Autodesk Inventor part; units mm, degrees
ref_plane "YZ Plane" through (0, 0, 0) normal (1, 0, 0) x (0, 1, 0)
ref_plane "XZ Plane" through (0, 0, 0) normal (0, 1, 0) x (-1, 0, 0)
ref_plane "XY Plane" through (0, 0, 0) normal (0, 0, 1) x (1, 0, 0)
sketch "Sketch1" plane through (0, 0, 0) normal (0, 1, 0) x (-1, 0, 0)
  line L0 (0, 0) -> (100, 0)
  line L1 (100, 0) -> (100, -100)
  line L2 (100, -100) -> (0, -100)
  line L3 (0, -100) -> (0, 0)
  dimension "d0" = 100
  dimension "d1" = 100
extrude "Extrusion1" add sketch "Sketch1" along normal blind 0.3
sketch "Sketch2" plane through (0, 0.3, 0) normal (0, 1, 0) x (1, 0, 0)
  line L0 (-100, 100) -> (-100, 0)
  line L1 (-100, 0) -> (0, 0)
  line L2 (0, 0) -> (0, 100)
  line L3 (0, 100) -> (-100, 100)
  line L4 (0, 0) -> (0, 50)
  line L5 (0, 0) -> (0, 100)
  line L6 (0, 50) -> (-50, 50)
  circle A0 centre (-50, 50) radius 1.5
  dimension "d4" = 50
  dimension "d5" = 3
extrude "Extrusion2" cut sketch "Sketch2" against normal blind 0.3 contours A0
sketch "Sketch3" plane through (0, 0.3, 0) normal (0, 1, 0) x (1, 0, 0)
  circle A0 centre (-50, 50) radius 1.5
  line L0 (-100, 100) -> (-100, 0)
  line L1 (-100, 0) -> (0, 0)
  line L2 (0, 0) -> (0, 100)
  line L3 (0, 100) -> (-100, 100)
  line L4 (-50, 50) -> (-57, 50)
  line L5 (-57, 47.5) -> (-57, 52.5) construction
  line L6 (-56.9, 47.5) -> (-56.9, 52.5)
  line L7 (-57.1, 52.5) -> (-57.1, 47.5)
  arc A1 (-57.1, 47.5) -> (-56.9, 47.5) centre (-57, 47.5) ccw
  arc A2 (-56.9, 52.5) -> (-57.1, 52.5) centre (-57, 52.5) ccw
  line L8 (-57, 50) -> (-65, 50)
  line L9 (-65, 47.5) -> (-65, 52.5) construction
  line L10 (-64.9, 47.5) -> (-64.9, 52.5)
  line L11 (-65.1, 52.5) -> (-65.1, 47.5)
  arc A3 (-65.1, 47.5) -> (-64.9, 47.5) centre (-65, 47.5) ccw
  arc A4 (-64.9, 52.5) -> (-65.1, 52.5) centre (-65, 52.5) ccw
  line L12 (-65, 50) -> (-77, 50)
  line L13 (-77, 47.5) -> (-77, 52.5) construction
  line L14 (-76.9, 47.5) -> (-76.9, 52.5)
  line L15 (-77.1, 52.5) -> (-77.1, 47.5)
  arc A5 (-77.1, 47.5) -> (-76.9, 47.5) centre (-77, 47.5) ccw
  arc A6 (-76.9, 52.5) -> (-77.1, 52.5) centre (-77, 52.5) ccw
  dimension "d8" = 7
  dimension "d9" = 2.5
  dimension "d10" = 0.2
  dimension "d11" = 8
  dimension "d12" = 2.5
  dimension "d13" = 0.2
  dimension "d14" = 12
  dimension "d15" = 2.5
  dimension "d16" = 0.2
extrude "Extrusion3" cut sketch "Sketch3" against normal blind 0.3 contours L14 A5 L15 A6 | L10 A3 L11 L12 L8 | L8 L12 L11 A4 L10 | L6 A1 L7 L8 L4 | L4 L8 L7 A2 L6
pattern_circular "Circular Pattern1" count 6 over 360 about axis through (-50, 0.3, -50) along (0, -1, 0) of "Extrusion3"
sketch "Sketch4" plane through (0, 0.3, 0) normal (0, 1, 0) x (1, 0, 0)
  line L0 (-51.3849, 42.6012) -> (-55.7151, 45.1012)
  arc A0 (-55.6151, 45.2744) -> (-55.7151, 45.1012) centre (-55.6651, 45.1878) ccw
  line L1 (-55.6151, 45.2744) -> (-51.2849, 42.7744)
  arc A1 (-51.3849, 42.6012) -> (-51.2849, 42.7744) centre (-51.3349, 42.6878) ccw
  line L2 (-55.3849, 35.673) -> (-59.7151, 38.173)
  arc A2 (-59.6151, 38.3462) -> (-59.7151, 38.173) centre (-59.6651, 38.2596) ccw
  line L3 (-59.6151, 38.3462) -> (-55.2849, 35.8462)
  arc A3 (-55.3849, 35.673) -> (-55.2849, 35.8462) centre (-55.3349, 35.7596) ccw
  arc A4 (-65.6151, 27.9539) -> (-65.7151, 27.7807) centre (-65.6651, 27.8673) ccw
  line L4 (-65.6151, 27.9539) -> (-61.2849, 25.4539)
  arc A5 (-61.3849, 25.2807) -> (-61.2849, 25.4539) centre (-61.3349, 25.3673) ccw
  line L5 (-61.3849, 25.2807) -> (-65.7151, 27.7807)
  line L6 (-44.2849, 45.1012) -> (-48.6151, 42.6012)
  arc A6 (-48.7151, 42.7744) -> (-48.6151, 42.6012) centre (-48.6651, 42.6878) ccw
  line L7 (-48.7151, 42.7744) -> (-44.3849, 45.2744)
  arc A7 (-44.2849, 45.1012) -> (-44.3849, 45.2744) centre (-44.3349, 45.1878) ccw
  line L8 (-40.2849, 38.173) -> (-44.6151, 35.673)
  arc A8 (-44.7151, 35.8462) -> (-44.6151, 35.673) centre (-44.6651, 35.7596) ccw
  line L9 (-44.7151, 35.8462) -> (-40.3849, 38.3462)
  arc A9 (-40.2849, 38.173) -> (-40.3849, 38.3462) centre (-40.3349, 38.2596) ccw
  arc A10 (-38.7151, 25.4539) -> (-38.6151, 25.2807) centre (-38.6651, 25.3673) ccw
  line L10 (-38.7151, 25.4539) -> (-34.3849, 27.9539)
  arc A11 (-34.2849, 27.7807) -> (-34.3849, 27.9539) centre (-34.3349, 27.8673) ccw
  line L11 (-34.2849, 27.7807) -> (-38.6151, 25.2807)
  line L12 (-42.9, 52.5) -> (-42.9, 47.5)
  arc A12 (-43.1, 47.5) -> (-42.9, 47.5) centre (-43, 47.5) ccw
  line L13 (-43.1, 47.5) -> (-43.1, 52.5)
  arc A13 (-42.9, 52.5) -> (-43.1, 52.5) centre (-43, 52.5) ccw
  line L14 (-34.9, 52.5) -> (-34.9, 47.5)
  arc A14 (-35.1, 47.5) -> (-34.9, 47.5) centre (-35, 47.5) ccw
  line L15 (-35.1, 47.5) -> (-35.1, 52.5)
  arc A15 (-34.9, 52.5) -> (-35.1, 52.5) centre (-35, 52.5) ccw
  arc A16 (-23.1, 47.5) -> (-22.9, 47.5) centre (-23, 47.5) ccw
  line L16 (-23.1, 47.5) -> (-23.1, 52.5)
  arc A17 (-22.9, 52.5) -> (-23.1, 52.5) centre (-23, 52.5) ccw
  line L17 (-22.9, 52.5) -> (-22.9, 47.5)
  line L18 (-48.6151, 57.3988) -> (-44.2849, 54.8988)
  arc A18 (-44.3849, 54.7256) -> (-44.2849, 54.8988) centre (-44.3349, 54.8122) ccw
  line L19 (-44.3849, 54.7256) -> (-48.7151, 57.2256)
  arc A19 (-48.6151, 57.3988) -> (-48.7151, 57.2256) centre (-48.6651, 57.3122) ccw
  line L20 (-44.6151, 64.327) -> (-40.2849, 61.827)
  arc A20 (-40.3849, 61.6538) -> (-40.2849, 61.827) centre (-40.3349, 61.7404) ccw
  line L21 (-40.3849, 61.6538) -> (-44.7151, 64.1538)
  arc A21 (-44.6151, 64.327) -> (-44.7151, 64.1538) centre (-44.6651, 64.2404) ccw
  arc A22 (-34.3849, 72.0461) -> (-34.2849, 72.2193) centre (-34.3349, 72.1327) ccw
  line L22 (-34.3849, 72.0461) -> (-38.7151, 74.5461)
  arc A23 (-38.6151, 74.7193) -> (-38.7151, 74.5461) centre (-38.6651, 74.6327) ccw
  line L23 (-38.6151, 74.7193) -> (-34.2849, 72.2193)
  line L24 (-55.7151, 54.8988) -> (-51.3849, 57.3988)
  arc A24 (-51.2849, 57.2256) -> (-51.3849, 57.3988) centre (-51.3349, 57.3122) ccw
  line L25 (-51.2849, 57.2256) -> (-55.6151, 54.7256)
  arc A25 (-55.7151, 54.8988) -> (-55.6151, 54.7256) centre (-55.6651, 54.8122) ccw
  line L26 (-59.7151, 61.827) -> (-55.3849, 64.327)
  arc A26 (-55.2849, 64.1538) -> (-55.3849, 64.327) centre (-55.3349, 64.2404) ccw
  line L27 (-55.2849, 64.1538) -> (-59.6151, 61.6538)
  arc A27 (-59.7151, 61.827) -> (-59.6151, 61.6538) centre (-59.6651, 61.7404) ccw
  arc A28 (-61.2849, 74.5461) -> (-61.3849, 74.7193) centre (-61.3349, 74.6327) ccw
  line L28 (-61.2849, 74.5461) -> (-65.6151, 72.0461)
  arc A29 (-65.7151, 72.2193) -> (-65.6151, 72.0461) centre (-65.6651, 72.1327) ccw
  line L29 (-65.7151, 72.2193) -> (-61.3849, 74.7193)
  line L30 (-57.1, 47.5) -> (-57.1, 52.5)
  arc A30 (-56.9, 52.5) -> (-57.1, 52.5) centre (-57, 52.5) ccw
  line L31 (-56.9, 52.5) -> (-56.9, 47.5)
  arc A31 (-57.1, 47.5) -> (-56.9, 47.5) centre (-57, 47.5) ccw
  line L32 (-65.1, 47.5) -> (-65.1, 52.5)
  arc A32 (-64.9, 52.5) -> (-65.1, 52.5) centre (-65, 52.5) ccw
  line L33 (-64.9, 52.5) -> (-64.9, 47.5)
  arc A33 (-65.1, 47.5) -> (-64.9, 47.5) centre (-65, 47.5) ccw
  arc A34 (-76.9, 52.5) -> (-77.1, 52.5) centre (-77, 52.5) ccw
  line L34 (-76.9, 52.5) -> (-76.9, 47.5)
  arc A35 (-77.1, 47.5) -> (-76.9, 47.5) centre (-77, 47.5) ccw
  line L35 (-77.1, 47.5) -> (-77.1, 52.5)
  circle A36 centre (-50, 50) radius 1.5
  line L36 (0, 0) -> (0, 100)
  line L37 (0, 100) -> (-100, 100)
  line L38 (-100, 100) -> (-100, 0)
  line L39 (-100, 0) -> (0, 0)
  line L40 (-76.9, 47.5) -> (-76.9, 52.5)
  line L41 (-76.9, 50) -> (-77, 50)
  line L42 (-76.9, 52.5) -> (-76.9, 47.5)
  line L43 (-77, 50) -> (-82, 50)
  line L44 (-87, 48) -> (-87, 52)
  line L45 (-87, 52) -> (-77, 52)
  line L46 (-77, 52) -> (-77, 48)
  line L47 (-77, 48) -> (-87, 48)
  line L48 (-87, 48) -> (-77, 52) construction
  line L49 (-87, 52) -> (-77, 48) construction
  circle A37 centre (-82, 50) radius 0.6
  line L50 (-82, 50) -> (-85.5, 50)
  circle A38 centre (-85.5, 50) radius 0.6
  circle A39 centre (-50, 50) radius 1.5
  line L51 (-50, 50) -> (-77, 50)
  circle A40 centre (-50, 50) radius 6
  line L52 (-50, 50) -> (-63.5, 50)
  line L53 (-50, 48) -> (-50, 52)
  line L54 (-50, 52) -> (-77, 52)
  line L55 (-77, 52) -> (-77, 48)
  line L56 (-77, 48) -> (-50, 48)
  line L57 (-50, 48) -> (-77, 52) construction
  line L58 (-50, 52) -> (-77, 48) construction
  dimension "d22" = 0.1
  dimension "d23" = 5
  dimension "d24" = 4
  dimension "d25" = 10
  dimension "d26" = 1.2
  dimension "d27" = 3.5
  dimension "d28" = 1.2
  dimension "d29" = 12
  dimension "d30" = 13.5
  dimension "d31" = 4
  dimension "d32" = 27
properties part number "layer_1"
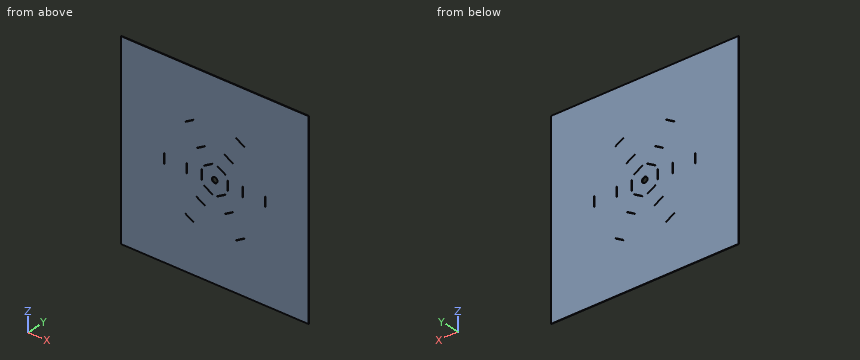
Part model, mm, in its own coordinate system. Coordinates: 2 decimals unless noted, no trailing zeros. Use a Markdown table: item, result.
(1) Cut at A-A on z = -50. State how many separate pieces and enclosed holes the cut face has, then the cut area to 3 significant figures.
A:
| item | result |
|---|---|
| separate pieces | 8 |
| enclosed holes | 0 |
| area | 28.7 mm^2 |
(2) Flat gauge pin, fed straight in: pin 1 (2.5 mm diameter, centred on x = -50, z = -50, fed in from +Y). Where does the tip first touch, or does it go through?
A:
| item | result |
|---|---|
| pin 1 | passes through |
(3) Probe L1, parallel to Z at x = -50, y = 0.25; L2, parallel to Z at x = -53.5, y = 0.2; L3, parallel to Z at x = -37, y = 0.1. List the from-to ranges inside material, lowest first.
A:
| item | result |
|---|---|
| L1 | z = -100 to -51.5, -48.5 to 0 |
| L2 | z = -100 to -56.18, -55.95 to -44.05, -43.82 to 0 |
| L3 | z = -100 to -73.79, -73.56 to -26.44, -26.21 to 0 |
